Geometry check sheet. Reference: the model listing, model coordinates, mm. Coordinates: 2 decimals unless noted, no trailing zeros. Loops run counter-clockwise (first coordinate to the right, second up) from the corner with the lowest first, then second, coordinate; pieces in that order, holes last. Notation, with made-up numbers: (-39, -6.5) -> (2, -6.5) arc R5 cw to (2, 2.5) -> close; hole circle Ø11 at (-8.75, -17.75). An arc over 180 degrees is marked (long way). Answer as a JSON object with one key per item and string values.
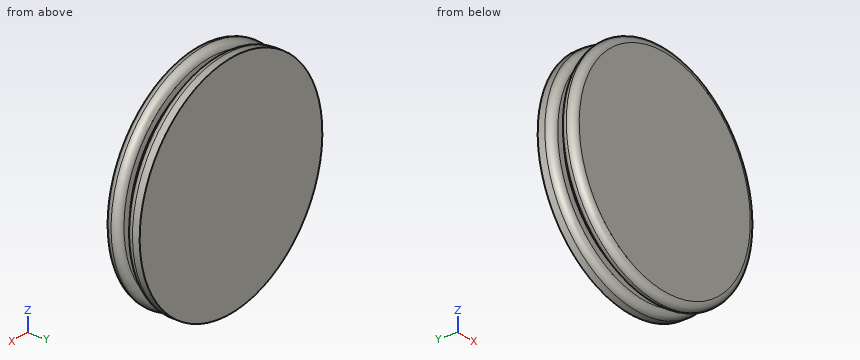
from build123d import *

# Parameters (mm, degrees)
SKETCH1_R           = 20
BOSS_EXTRUDE1_DEPTH = 2.54
SKETCH2_R           = 17.5
BOSS_EXTRUDE2_DEPTH = 1.27
SKETCH3_R           = 20
BOSS_EXTRUDE3_DEPTH = 2.54
FILLET1_R           = 1.27
FILLET2_R           = 1.27


with BuildPart() as part:
    # Sketch1 → Boss-Extrude1 (new body)
    with BuildSketch(Plane(origin=(0, 0, 0), x_dir=(1, 0, 0), z_dir=(0, 1, 0))):
        with Locations(Location((0, 0, 0), (0, 0, 270))):
            Circle(SKETCH1_R)
    extrude(amount=BOSS_EXTRUDE1_DEPTH)

    # Sketch2 → Boss-Extrude2 (add)
    with BuildSketch(Plane(origin=(0, 2.54, 0), x_dir=(1, 0, 0), z_dir=(0, 1, 0))):
        with Locations(Location((0, 0, 0), (0, 0, 270))):
            Circle(SKETCH2_R)
    extrude(amount=BOSS_EXTRUDE2_DEPTH)

    # Sketch3 → Boss-Extrude3 (add)
    with BuildSketch(Plane(origin=(0, 3.81, 0), x_dir=(1, 0, 0), z_dir=(0, 1, 0))):
        with Locations(Location((0, 0, 0), (0, 0, 270))):
            Circle(SKETCH3_R)
    extrude(amount=BOSS_EXTRUDE3_DEPTH)

    # Fillet1
    fillet1_edges = [part.edges().sort_by_distance(p)[0] for p in [
        (0, 3.81, -20),
    ]]
    fillet(fillet1_edges, radius=FILLET1_R)

    # Fillet2
    fillet2_edges = [part.edges().sort_by_distance(p)[0] for p in [
        (0, 0, -20),
        (0, 2.54, -20),
    ]]
    fillet(fillet2_edges, radius=FILLET2_R - 0.0001)  # a hair under: the kernel refuses the full size


solid = part.part
1. Section check C-C, the plane y = 3. Record the boundary of the cut face in (x, z).
Evaluation:
{"outline": "circle Ø35 at (0, 0)"}
2. Thickness scan on probe 1 along Y at (x, z) = (11.5, -15); probe 2 along Z at (x, y) = (17.5, 2); probe 3 along X at (y, z) = (6, -5). Record the ranges inside material, lowest first. Write a range as from..to.
Evaluation:
{"probe 1": "y = 0.01..2.53, 3.82..6.35", "probe 2": "z = -9.2..9.2", "probe 3": "x = -19.36..19.36"}
3. Section check D-D, the plane y = 0.5. Record the boundary of the cut face in (x, z).
Evaluation:
{"outline": "circle Ø39.48 at (0, 0)"}
4. Depth check by flat-ended pin: P1, Ø18.5, axis at x = -8.5, z = -8, coming from the -Y side. Enter the tip coordinate at first touch or a pass-through.
Evaluation:
{"P1": "stops at y = 0"}
